For this review, take the finished solid that the model builds, in its own axes (mm). A direction names the side the tool comes from. Round coordinates to 2 decimals unless told otherwise and drop trailing zeros. Order: outer loops, then holes, each group sorted by start corner. A loop starts at its lowest first (then second) coordinate and runs counter-clockwise, first axis right, second up. Notation, with made-up numbers: (51.5, 68.5) -> (60.5, 68.5) arc R17 ccw to (60.5, 76.5) -> close; hole circle Ø9 at (64, 39). An arc over 180 degrees is marked (long way). Use a Markdown table: item, result. Add a question column.
1) Machinability: for faces 1 (the face through (232, 11, -25)), 2 (the face through (27.5, 6, -12)), 3 (the face through (456, 12, -12)), which of the approach directions +Z, -Z, +X, -X, +Y, -Y give a long, thin tool a straight path to every point of the face, cutting with its end or side? Answer none if there is none.
2) Consider section B-B (y = 4.5). State the section outline as (x, z) points, plus the area to 3 significant figures.
3) Consider section A-A (z = -8.5). State the section outline as (x, y) points, plus the area to 3 significant figures.
4) Wall thickness on line 1 along X through (y, z) = (4.25, -7): over which ranges is the line inside the solid? List them lowest first. Write a range as [from, to].
5) Clearance check with flat-ended pins moving along their axes: P1, Ø13, axis at y = 8, z = -18, coming from the +X side; P2, Ø10, axis at y = 2.5, z = -19.5, coming from the +X side; P3, Ø7.5, axis at x = 450, z = -17, coming from the -Y side. State where each tip first meets the part, or that it passes through.
```python
from build123d import *

# Parameters (mm, degrees)
SKETCH_1_W          = 470
SKETCH_1_H          = 25
EXTRUDE_1_DEPTH     = 22
SKETCH_2_W          = 27.5
SKETCH_2_H          = 12
CUT_EXTRUDE_1_DEPTH = 472.178310197
SKETCH_3_W          = 27.5
SKETCH_3_H          = 12
CUT_EXTRUDE_2_DEPTH = 472.178310197


with BuildPart() as part:
    # Эскиз1 → Бобышка-Вытянуть1 (new body)
    with BuildSketch(Plane(origin=(0, 0, 0), x_dir=(1, 0, 0), z_dir=(0, 1, 0))):
        with Locations((235, 12.5)):
            Rectangle(SKETCH_1_W, SKETCH_1_H)
    extrude(amount=EXTRUDE_1_DEPTH)

    # Эскиз2 → Вырез-Вытянуть1 (cut, through all)
    with BuildSketch(Plane.XY):
        with Locations((456.25, 6)):
            Rectangle(SKETCH_2_W, SKETCH_2_H)
    extrude(amount=-CUT_EXTRUDE_1_DEPTH, mode=Mode.SUBTRACT)

    # Эскиз3 → Вырез-Вытянуть2 (cut, through all)
    with BuildSketch(Plane.XY):
        with Locations((13.75, 6)):
            Rectangle(SKETCH_3_W, SKETCH_3_H)
    extrude(amount=-CUT_EXTRUDE_2_DEPTH, mode=Mode.SUBTRACT)


solid = part.part
```
Results list:
| question | item | result |
|---|---|---|
| 1 | face 1 | -Z, +X, -X, +Y, -Y |
| 1 | face 2 | +Z, -Z, -X, -Y |
| 1 | face 3 | +Z, -Z, +X, -Y |
| 2 | outline | (27.5, -25) -> (442.5, -25) -> (442.5, 0) -> (27.5, 0) -> close |
| 2 | area | 10,400 mm2 |
| 3 | outline | (0, 12) -> (27.5, 12) -> (27.5, 0) -> (442.5, 0) -> (442.5, 12) -> (470, 12) -> (470, 22) -> (0, 22) -> close |
| 3 | area | 9,680 mm2 |
| 4 | line 1 | [27.5, 442.5] |
| 5 | P1 | x = 470 |
| 5 | P2 | x = 442.5 |
| 5 | P3 | y = 12 |
